Solid Edge part; units mm, degrees
sketch "Sketch1" plane through (0, 0, 8) normal (0, 0, 1) x (1, 0, 0)
  line L0 (-28, -49) -> (28, -49)
  line L1 (28, -49) -> (28, 24)
  line L2 (28, 24) -> (-28, 24)
  line L3 (-28, 24) -> (-28, -49)
  circle A0 centre (0, 0) radius 12
  circle A1 centre (11.3137, 11.3137) radius 1.7
  circle A2 centre (-11.3137, 11.3137) radius 1.7
  circle A3 centre (-11.3137, -11.3137) radius 1.7
  circle A4 centre (11.3137, -11.3137) radius 1.7
extrude "ExtrudedProtrusion_1" add sketch "Sketch1" along normal blind 4
sketch "Sketch2" plane through (0, 0, 12) normal (0, 0, 1) x (1, 0, 0)
  line L0 (22, -49) -> (28, -49)
  line L1 (28, -49) -> (28, 24)
  line L2 (28, 24) -> (22, 24)
  line L3 (22, 24) -> (22, -49)
extrude "ExtrudedProtrusion_2" add sketch "Sketch2" along normal blind 56
sketch "Sketch3" plane through (22, 0, 0) normal (1, 0, 0) x (0, 1, 0)
  circle A0 centre (-43, 63) radius 1.7
  circle A1 centre (-43, 17) radius 1.7
  circle A2 centre (18, 63) radius 1.7
  circle A3 centre (18, 17) radius 1.7
extrude "ExtrudedCutout_1" cut sketch "Sketch3" along normal blind 6
Geometry check sheet. Reference: the model listing, model coordinates, mm. A direction names the side the tool comes from. Round coordinates to 2 decimals unless told otherwise and drop trailing zeros. Order: outer loops, then holes, each group sorted by start corner. A loop starts at its lowest first (then second) coordinate and runs counter-clockwise, first axis right, second up. Notation, with made-up numbers: M -0.75,77.25 L 44.25,77.25 A27 ccw 44.25,101.25 Z; hole C 33,-2 d4. An arc over 180 degrees is marked long. Answer in a Markdown table with one row per item. Add a question column.
Item 1: Sectioned sample at D-D, the plane y = -14. Enter the section's corners in (x, z), plus the area to 3 significant figures.
Item 2: Depth check by flat-ended pin: pin 1 Ø10 at (y, z) = (-6, 56) entering from -X; pin 2 Ø2 at (x, y) = (5, -19.5) entering from +Z. Enter the tip coordinate at first touch or a pass-through.
Item 3: Set-up check for faces 1 (the face through (25, -12, 68)), 2 (the face through (22, -12, 40)): record each of +Z, -Z, +X, -X, +Y, -Y from which the full face is reachable in a straight line by a thin tool's end or side.
Item 4: Material ranges on L1, parallel to Z at x = 24.25, y = -43; L2, parallel to Y at x = 0, z = 10.05; L3, parallel to Z at x = 23, y = -43.5, recorded low to high. Write a range as [from, to].
Item 5: Draft check along Y on faces 3 (the face through (24.958, 18.914, 61.567)), 4 (the face through (24.96, -44.7, 16.93)), 5 (the face through (28, -13, 38)), 6 (the face through (23, 24, 29)). Enter one of: released by +Y, released by -Y, zero draft, split by the parting line, or undercut.
Item 6: Sectioned sample at B-B, the plane y = -43. Enter the section's corners in (x, z).
Item 7: Sectioned sample at C-C, the plane y = 0. Enter the section's corners in (x, z), plus the area to 3 significant figures.
Item 8: Sectioned sample at A-A, the plane x = 0. Enter the section's corners in (y, z).
Filled in:
| question | item | result |
|---|---|---|
| 1 | outline | M -28,8 L 28,8 L 28,68 L 22,68 L 22,12 L -28,12 Z |
| 1 | area | 560 mm² |
| 2 | pin 1 | stops at x = 22 |
| 2 | pin 2 | stops at z = 12 |
| 3 | face 1 | +Z, +X, -X, +Y, -Y |
| 3 | face 2 | +Z, -X, +Y, -Y |
| 4 | L1 | z = [8, 15.3], [18.7, 61.3], [64.7, 68] |
| 4 | L2 | y = [-49, -12], [12, 24] |
| 4 | L3 | z = [8, 15.38], [18.62, 61.38], [64.62, 68] |
| 5 | face 3 | undercut |
| 5 | face 4 | undercut |
| 5 | face 5 | zero draft |
| 5 | face 6 | released by +Y |
| 6 | outline | M -28,8 L 28,8 L 28,15.3 L 22,15.3 L 22,12 L -28,12 Z; M 22,18.7 L 28,18.7 L 28,61.3 L 22,61.3 Z; M 22,64.7 L 28,64.7 L 28,68 L 22,68 Z |
| 7 | outline | M -28,8 L -12,8 L -12,12 L -28,12 Z; M 12,8 L 28,8 L 28,68 L 22,68 L 22,12 L 12,12 Z |
| 7 | area | 464 mm² |
| 8 | outline | M -49,8 L -12,8 L -12,12 L -49,12 Z; M 12,8 L 24,8 L 24,12 L 12,12 Z |
